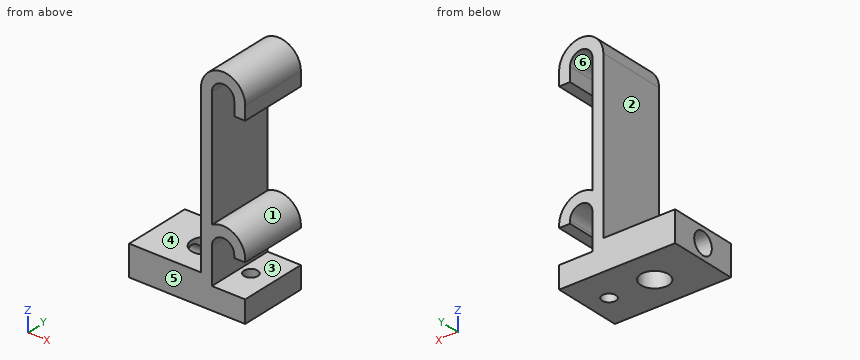
from build123d import *

# Parameters (mm, degrees)
F1_DEPTH = 25
F2_R     = 5
F3_DEPTH = 25
F4_R     = 2.5
F5_DEPTH = 15
F6_R     = 3.95
F7_DEPTH = 17


with BuildPart() as f1:
    # F0 (on Front) → F1 (new body)
    with BuildSketch(Plane.XZ):
        with BuildLine():
            ThreePointArc((-4.05, 0), (0, 4.05), (4.05, 0))
            Line((4.05, 0), (4.05, -5))
            Line((4.05, -5), (8, -5))
            Line((8, -5), (8, 0))
            ThreePointArc((8, 0), (0, 8), (-8, 0))
            Line((-8, 0), (-8, -50))
            Line((-8, -50), (-8, -60))
            Line((-8, -60), (-34, -60))
            Line((-34, -60), (-34, -71))
            Line((-34, -71), (-4.05, -71))
            Line((-4.05, -71), (7.991412, -71))
            Line((7.991412, -71), (7.991412, -63))
            Line((7.991412, -63), (-4.05, -63))
            Line((-4.05, -63), (-4.05, -50))
            ThreePointArc((-4.05, -50), (0, -45.95), (4.05, -50))
            Line((4.05, -50), (4.05, -51))
            Line((4.05, -51), (7.991412, -51))
            Line((7.991412, -51), (7.999683, -50.071239))
            ThreePointArc((7.999683, -50.071239), (4.005794, -43.075145), (-4.05, -43.100906))
            Line((-4.05, -43.100906), (-4.05, 0))
        make_face()
    extrude(amount=F1_DEPTH)

    # F2 (on face) → F3 (cut)
    with BuildSketch(Plane.XY.offset(-60)):
        with Locations((-16.5, -12.5)):
            Circle(F2_R)
    extrude(amount=-F3_DEPTH, mode=Mode.SUBTRACT)

    # F4 (on face) → F5 (cut)
    with BuildSketch(Plane(origin=(0, 0, -71), x_dir=(1, 0, 0), z_dir=(0, 0, -1))):
        with Locations((0, 12.5)):
            Circle(F4_R)
    extrude(amount=-F5_DEPTH, mode=Mode.SUBTRACT)

    # F6 (on face) → F7 (cut)
    with BuildSketch(Plane(origin=(-34, 0, 0), x_dir=(0, -1, 0), z_dir=(-1, 0, 0))):
        with Locations((12.5, -65.5)):
            Circle(F6_R)
    extrude(amount=-F7_DEPTH, mode=Mode.SUBTRACT)


solid = f1.part
Work out the finished part from the listing and answer in its coordinate system (mm). Face numbers are marked on the shaded views. A direction names the side the tool comes from. Round coordinates to 2 decimals unless told otherwise and drop trailing zeros. Loops run counter-clockwise (first coordinate to the right, second up) from the corner with the lowest first, then second, coordinate; pieces in that order, holes last. Notation, with made-up numbers: (61.25, 36.5) - (65.25, 36.5) arc R23 cw to (65.25, 68.5) - close; hole circle Ø10 at (51, -18). An arc over 180 degrees is marked (long way). Use one line per item in the form item = value. Start each with the question number.
(1) Find section B-B on z = -65.5. Determine the outline of the cut face in (x, y), and give its area (3 significant figures).
(2) Consider line 1 (X direction, y = -12.5, z = -63.5); line 2 (Y direction, x = 0, z = -65.75); line 3 (Z direction, x = -24.25, y = -12.5). Determine where each line is inside the solid, lowest interval first.
(3) Find section A-A on x = 0. Determine the outline of the cut face in (y, z).
(4) Determine the mould class of the marked faces 1, 2 and 3 for opening direction X: +X half, -X half, draft (parallel to the pull), parting line (faces both ways), or undercut.
(5) Find section C-C on y = -18.5. Determine the outline of the cut face in (x, z).
(6) Find section D-D on y = -11. Give the number of separate pieces and of enclosed holes in the cut face, and give its area (3 significant figures).
(7) Flat-ended cylindrical pins translate along their axes: P1, Ø12, axis at x = -28, y = -6.5, coming from the +Z side; P2, Ø6.5, axis at y = -10, z = -58.5, coming from the +X side; P3, Ø5.5, axis at y = -15, z = -1.5, coming from the -X side; P4, Ø6, axis at x = -16.5, y = -12.5, coming from the -Z side. Find the tip coordinate at first contact, or state that the pin passes through.
(8) Which of the six approach directions +Z, -Z, +X, -X, +Y, -Y give full straight-line access (tool end or side, diameter ignored) to the marked faces 4, 5 and 6?
Answer list:
q1.outline = (-34, -25) - (7.99, -25) - (7.99, 0) - (-34, 0) - (-34, -8.55) - (-19.57, -8.55) arc R5 cw (long way) to (-19.57, -16.45) - (-34, -16.45) - close; hole circle Ø5 at (0, -12.5)
q1.area = 848 mm^2
q2.line_1 = -11.5 to -2.5, 2.5 to 7.99
q2.line_2 = -25 to -15, -10 to 0
q2.line_3 = -71 to -69.45, -61.55 to -60
q3.outline = (-25, -71) - (-15, -71) - (-15, -63) - (-25, -63) - close; (-25, -45.95) - (0, -45.95) - (0, -42) - (-25, -42) - close; (-25, 4.05) - (0, 4.05) - (0, 8) - (-25, 8) - close; (-10, -71) - (0, -71) - (0, -63) - (-10, -63) - close
q4.face_1 = undercut
q4.face_2 = -X half
q4.face_3 = draft
q5.outline = (-34, -71) - (7.99, -71) - (7.99, -63) - (-4.05, -63) - (-4.05, -50) arc R4.05 cw to (4.05, -50) - (4.05, -51) - (7.99, -51) - (8, -50.07) arc R8 ccw to (-4.05, -43.1) - (-4.05, 0) arc R4.05 cw to (4.05, 0) - (4.05, -5) - (8, -5) - (8, 0) arc R8 ccw to (-8, 0) - (-8, -60) - (-34, -60) - close
q6.separate_pieces = 4
q6.enclosed_holes = 0
q6.area = 587 mm^2
q7.P1 = -60
q7.P2 = -4.05
q7.P3 = -8
q7.P4 = through
q8.face_4 = +Z, -X, +Y, -Y
q8.face_5 = +Z, -Z, +X, -X, -Y
q8.face_6 = +Y, -Y
